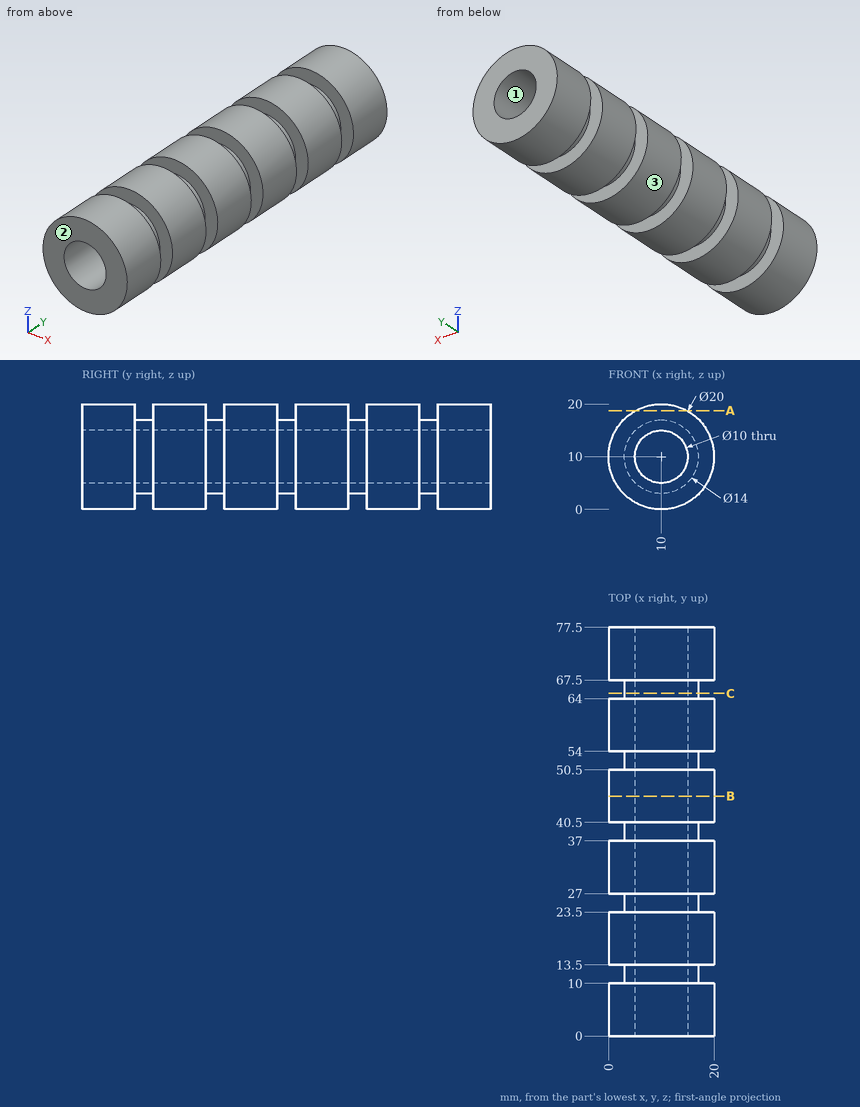
Study the drawing (mm; zero at the part's minimum x, y, z) and answer. Give positions to 0.01 mm unless a question says otherwise; leave off trailing zeros. Order: outer loops, then holes, each group sorted by start corner. A loop starts at its lowest first (then second) coordinate and runs counter-clockwise, first axis right, second up. Notation, with made-up numbers: (-23, 71.25) - (16, 71.25) arc R31 ccw to (16, 103.25) - close; hole circle Ø1 at (16.25, 15.25). An arc over 180 degrees is marked (long way). Answer in a Markdown table with one row per item. Add a question column.
Q1. Find the intervals of material crossed by line 1 along Y through (x, z) = (4, 5.5); line 2 along X through (y, z) = (56.5, 10); line 3 along X through (y, z) = (26, 10), in increasing order. Write a range as [from, to].
Q2. Given P1, Ø12, axis at x = 16.5, z = 10.5, coming from the -Y side; P2, Ø1, axis at x = 17, y = 21, coming from the +Z side; P3, Ø3, axis at x = 16.5, y = 49.5, coming from the -Z side; P4, Ø8, axis at y = 62, z = 17.5, coming from the +X side, each flat-ended and moving along its own axis, determine where each tip first touches the part or whether it passes through.
Q3. For a pull along Z with two mould halves and no side action, classify the marked faces 1, 2 and 3 as released by +Z, released by -Z, zero draft, split by the parting line, or undercut.
Q4. The part is cut by section A-A (z = 18.75). Determine the outline of the cut face in (x, y).
Q5. The part is cut by section B-B (y = 45.5). Determine the outline of the cut face in (x, z).
Q6. The part is cut by section C-C (y = 65). Determine the outline of the cut face in (x, z).
Determined:
| question | item | result |
|---|---|---|
| 1 | line 1 | y = [0, 10], [13.5, 23.5], [27, 37], [40.5, 50.5], [54, 64], [67.5, 77.5] |
| 1 | line 2 | x = [0, 5], [15, 20] |
| 1 | line 3 | x = [3, 5], [15, 17] |
| 2 | P1 | stops at y = 0 |
| 2 | P2 | stops at z = 17.6 |
| 2 | P3 | stops at z = 1.34 |
| 2 | P4 | stops at x = 19.37 |
| 3 | face 1 | undercut |
| 3 | face 2 | zero draft |
| 3 | face 3 | split by the parting line |
| 4 | outline | (5.16, 0) - (14.84, 0) - (14.84, 10) - (5.16, 10) - close; (5.16, 13.5) - (14.84, 13.5) - (14.84, 23.5) - (5.16, 23.5) - close; (5.16, 27) - (14.84, 27) - (14.84, 37) - (5.16, 37) - close; (5.16, 40.5) - (14.84, 40.5) - (14.84, 50.5) - (5.16, 50.5) - close; (5.16, 54) - (14.84, 54) - (14.84, 64) - (5.16, 64) - close; (5.16, 67.5) - (14.84, 67.5) - (14.84, 77.5) - (5.16, 77.5) - close |
| 5 | outline | circle Ø20 at (10, 10); hole circle Ø10 at (10, 10) |
| 6 | outline | circle Ø14 at (10, 10); hole circle Ø10 at (10, 10) |
